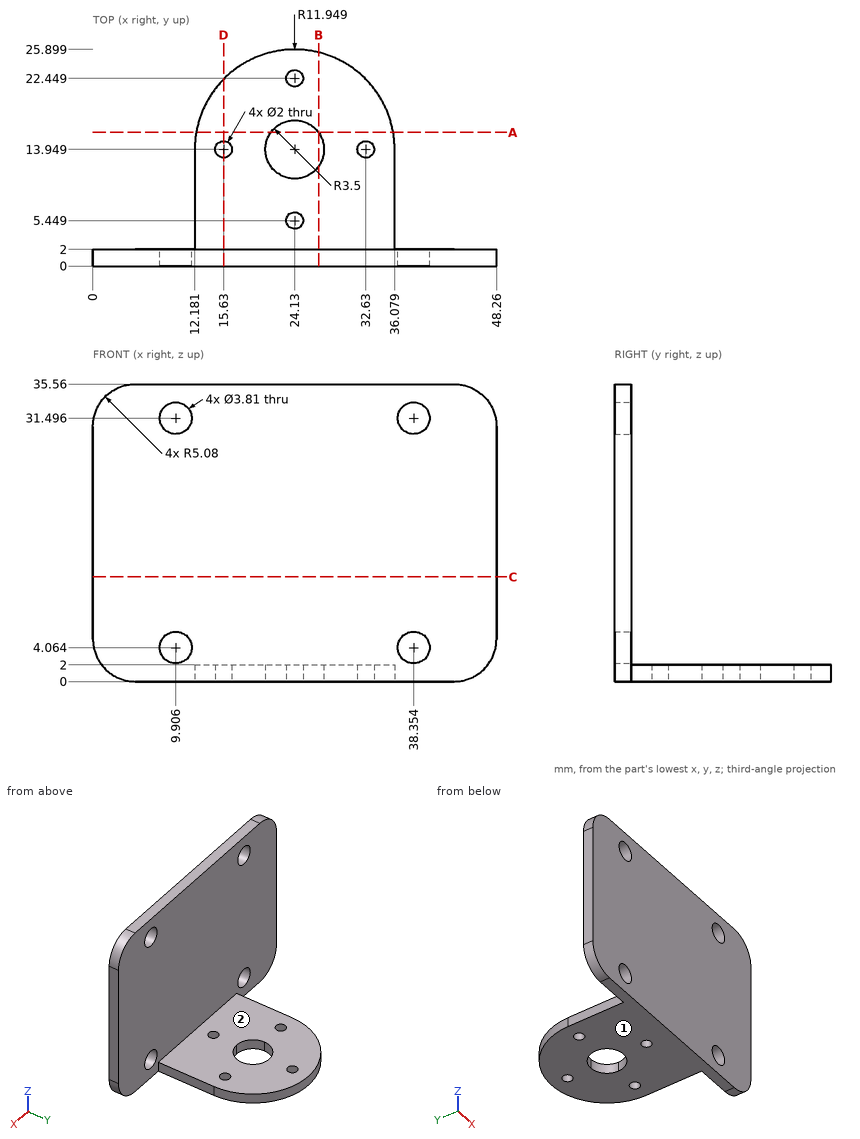
For this review, use the dimensioned drawing (mm, ordinates from the lowest corner) and the shaded views. A direction names the side the tool comes from. Coordinates: 2 decimals unless noted, no trailing zeros. Write each loop counter-clockwise with the first axis right and the second up, starting at its lowest first coordinate (ties: lowest second). Pieces come first, ordered by that corner, then holes. Notation, with made-up numbers: (-24, -17) -> (7, -17) arc R24 ccw to (7, 15) -> close; hole circle Ø7 at (-20.5, 64.5). An arc over 180 degrees is marked (long way). Write each question's results on one line, items separated by ' | '. Start each with the question number.
(1) Take a section at B-B on x = 27. Write out the cut boundary in (y, z).
(2) Take a section at D-D on x = 15.63. Write out the cut boundary in (y, z), and give its area (3 significant figures).
(3) Clearance check with flat-ended pins moving along their axes: P1, Ø4.5, axis at x = 38.354, z = 4.064, coming from the +Y side; P2, Ø2.5, axis at x = 15.63, y = 13.95, coming from the +Z side; P3, Ø1.6, axis at y = 10.5, z = 1, coming from the +X side; P4, Ø3, axis at x = 9.906, z = 4.064, coming from the -Y side. State where each tip first meets the part, or that it passes through.
(4) Take a section at A-A on y = 16. Write out the cut boundary in (x, z).
(5) For line 1 along Y through (x, z) = (33.5, 14); line 2 along Y through (x, z) = (32.63, 1.05), list the stretches that pass through material, from the lowest coordinate up. Write a range as from..to.
(6) Take a section at C-C on z = 12.5. Write out the cut boundary in (x, y).
(7) Tool access review of the marked faces 1 and 2: name each direction out of +Z, -Z, +X, -X, +Y, -Y from which nothing blocks a thin tool from reaching the whole face with its end or side.
Results found:
1) outline: (0, 0) -> (11.95, 0) -> (11.95, 2) -> (2, 2) -> (2, 35.56) -> (0, 35.56) -> close; (15.95, 0) -> (25.55, 0) -> (25.55, 2) -> (15.95, 2) -> close
2) outline: (0, 0) -> (12.95, 0) -> (12.95, 2) -> (2, 2) -> (2, 35.56) -> (0, 35.56) -> close; (14.95, 0) -> (22.35, 0) -> (22.35, 2) -> (14.95, 2) -> close | area: 108 mm2
3) P1: stops at y = 2 | P2: stops at z = 2 | P3: stops at x = 36.08 | P4: passes through
4) outline: (12.36, 0) -> (21.29, 0) -> (21.29, 2) -> (12.36, 2) -> close; (26.97, 0) -> (35.9, 0) -> (35.9, 2) -> (26.97, 2) -> close
5) line 1: y = 0..2 | line 2: y = 0..12.95, 14.95..22.35
6) outline: (0, 0) -> (48.26, 0) -> (48.26, 2) -> (0, 2) -> close
7) face 1: -Z, +X, -X, +Y, -Y | face 2: +Z, +X, -X, +Y
